from build123d import *

# Parameters (mm, degrees)
F0_R      = 5.5
F1_DEPTH  = 5
F1_FACE_R = 5.5
F2_DEPTH  = 1.5
F2_TAPER  = -45
F3_R      = 0.2
F4_R      = 1.75
F5_DEPTH  = 6.501
F4_R_2    = 3
F6_DEPTH  = 3.5


with BuildPart() as f1:
    # F0 (on Top) → F1 (new body)
    with BuildSketch(Plane.XY):
        Circle(F0_R)
    extrude(amount=F1_DEPTH)

    # F1_face (on face) → F2 (join)
    with BuildSketch(Plane.XY.offset(5)):
        Circle(F1_FACE_R)
    extrude(amount=F2_DEPTH, taper=F2_TAPER)

    # F3
    f3_edges = [f1.edges().sort_by_distance(p)[0] for p in [
        (-7, 0, 6.5),
    ]]
    fillet(f3_edges, radius=F3_R)

    # F4 (on face) → F5 (cut, through all)
    with BuildSketch(Plane.XY.offset(6.5)):
        Circle(F4_R)
    extrude(amount=-F5_DEPTH, mode=Mode.SUBTRACT)

    # F4 (on face) → F6 (cut)
    with BuildSketch(Plane.XY.offset(6.5)):
        Circle(F4_R_2)
        Circle(F4_R, mode=Mode.SUBTRACT)
    extrude(amount=-F6_DEPTH, mode=Mode.SUBTRACT)


solid = f1.part
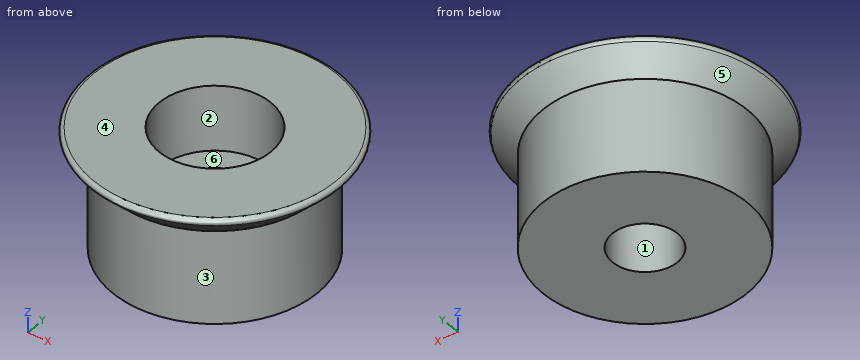
The listing builds one solid part. Answer for the finished solid, in the listing's coordinates (mm). Face numbers are marked on the shaded views. A direction names the side the tool comes from. Coordinates: 2 decimals unless noted, no trailing zeros. Loops run counter-clockwise (first coordinate to the right, second up) from the corner with the lowest first, then second, coordinate; pieces in that order, holes last. Notation, with made-up numbers: (-39, 26) -> (19, 26) arc R37 ccw to (19, 64) -> close; hole circle Ø7 at (89, 53.25). An arc over 180 degrees is marked (long way). Answer in a Markdown table with one row per item. Add a question column.
1. Consider line 1 (Y direction, x = 0, z = 2.3); line 2 (Y direction, x = 0, z = 4.35); line 3 (X direction, y = 0.75, z = 5.25). Determine where each line is inside the solid, lowest interval first. Write a range as [from, to].
2. The part is cut by section A-A, the plane x = 0. Write down the section's boundary in (y, z), then the cut area to 3 significant figures.
3. For the marked faces 1, 2 and 3, determine the directions among +Z, -Z, +X, -X, +Y, -Y from which every point of the face is accessible in a straight line to the end or side of a thin tool.
4. Flat-ended cylindrical pins translate along their axes: P1, Ø1, axis at y = 5, z = 4.5, coming from the +X side; P2, Ø4, axis at x = 0, y = 0, coming from the +Z side; P3, Ø1.5, axis at x = -2, z = 1.5, coming from the -Y side. Find the tip coordinate at first contact, or state that the pin passes through.
5. The part is cut by section B-B, the plane z = 2.75. Write down the section's boundary in (x, y).
6. The part is cut by section C-C, the plane z = 4. Write down the section's boundary in (x, y).
7. Determine the mould class of the marked faces 4, 5 and 6 for opening direction Y: +Y half, -Y half, draft (parallel to the pull), parting line (faces both ways), or undercut.
Answer below:
| question | item | result |
|---|---|---|
| 1 | line 1 | [-5.5, -1.75], [1.75, 5.5] |
| 1 | line 2 | [-5.5, -3], [3, 5.5] |
| 1 | line 3 | [-5.7, -2.9], [2.9, 5.7] |
| 2 | outline | (-6.66, 6.16) -> (-5.5, 5) -> (-5.5, 0) -> (-1.75, 0) -> (-1.75, 3) -> (-3, 3) -> (-3, 6.5) -> (-6.52, 6.5) arc R0.2 ccw to start; (1.75, 0) -> (5.5, 0) -> (5.5, 5) -> (6.66, 6.16) arc R0.2 ccw to (6.52, 6.5) -> (3, 6.5) -> (3, 3) -> (1.75, 3) -> close |
| 2 | area | 42.2 mm2 |
| 3 | face 1 | +Z, -Z |
| 3 | face 2 | +Z |
| 3 | face 3 | -Z |
| 4 | P1 | x = 3.16 |
| 4 | P2 | z = 3 |
| 4 | P3 | y = -5.36 |
| 5 | outline | circle Ø11 at (0, 0); hole circle Ø3.5 at (0, 0) |
| 6 | outline | circle Ø11 at (0, 0); hole circle Ø6 at (0, 0) |
| 7 | face 4 | draft |
| 7 | face 5 | parting line |
| 7 | face 6 | undercut |
